Verification items for the finished model (mm, model axes). Give positions to 0.01 mm unless a question says otherwise; leave off trailing zeros. Loops run counter-clockwise (first coordinate to the right, second up) from the corner with the lowest first, then second, coordinate; pieces in that order, holes last. Notation, with made-up numbers: (-37, 87.5) - (-33, 87.5) arc R19 ccw to (-33, 93.5) - close; hole circle Ø3 at (-32.75, 37.5). An arc over 180 degrees is marked (long way). One line per question, with ' | ' between items. Start each with the question number.
1. Thickness scan on line 1 along Y through (x, z) = (10, 21.5); line 2 along X through (y, z) = (-21.5, 8.75); line 3 along Z through (x, y) = (-13, -6). Record the ranges inside material, lowest first. Write a range as from..to.
2. Section check C-C, the plane y = -23.5. Enter the section's corners in (x, z), then the cut area to 3 significant figures.
3. Section check B-B, the plane z = 16. Enter the section's corners in (x, y).
4. Depth check by flat-ended pin: pin 1 Ø5 at (y, z) = (0, 22.5) entering from -X. Enter the tip coordinate at first touch or a pass-through.
5. Section check A-A, the plane x = 11. Enter the section's corners in (y, z), then the cut area to 3 significant figures.
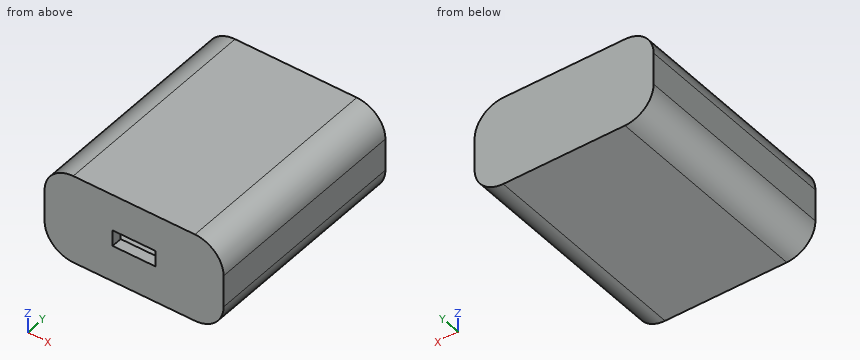
from build123d import *

# Parameters (mm, degrees)
F0_W     = 50
F0_H     = 60
F1_DEPTH = 25
F2_R     = 8
F3_T     = -3
F4_W     = 12
F4_H     = 4.5
F5_DEPTH = 3


with BuildPart() as f1:
    # F0 (on Top) → F1 (new body)
    with BuildSketch(Plane.XY):
        Rectangle(F0_W, F0_H)
    extrude(amount=F1_DEPTH)

    # F2
    f2_edges = [f1.edges().sort_by_distance(p)[0] for p in [
        (25, 0, 25),
        (25, 0, 0),
        (-25, 0, 0),
        (-25, 0, 25),
    ]]
    fillet(f2_edges, radius=F2_R)

    # F3 (hollow: no face is removed)
    offset(amount=F3_T, mode=Mode.SUBTRACT)

    # F4 (on face) → F5 (cut)
    with BuildSketch(Plane.XZ.offset(30)):
        with Locations((0, 12.5)):
            Rectangle(F4_W, F4_H)
    extrude(amount=-F5_DEPTH, mode=Mode.SUBTRACT)


solid = f1.part
Results list:
1) line 1: -30..-27, 27..30 | line 2: -25..-22, 22..25 | line 3: 0..3, 22..25
2) outline: (-25, 8) arc R8 ccw to (-17, 0) - (17, 0) arc R8 ccw to (25, 8) - (25, 17) arc R8 ccw to (17, 25) - (-17, 25) arc R8 ccw to (-25, 17) - close; hole (-22, 8) arc R5 ccw to (-17, 3) - (17, 3) arc R5 ccw to (22, 8) - (22, 17) arc R5 ccw to (17, 22) - (-17, 22) arc R5 ccw to (-22, 17) - close | area: 381 mm²
3) outline: (-25, -30) - (25, -30) - (25, 30) - (-25, 30) - close; hole (-22, -27) - (22, -27) - (22, 27) - (-22, 27) - close
4) pin 1: x = -24.42
5) outline: (-30, 0) - (30, 0) - (30, 25) - (-30, 25) - close; hole (-27, 3) - (27, 3) - (27, 22) - (-27, 22) - close | area: 474 mm²
